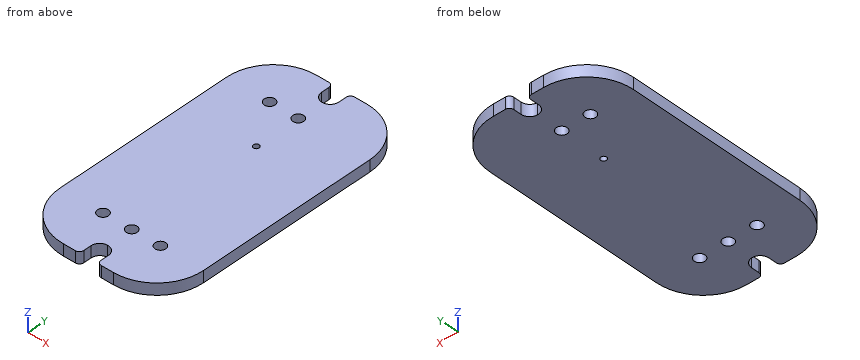
```python
from build123d import *

# Parameters (mm, degrees)
BOARD_DEPTH            = 0.8
SKETCH2_R              = 0.375
NON_PLATED_HOLES_DEPTH = 11.765221781
SKETCH3_R              = 0.2
PLATED_HOLES_DEPTH     = 11.765221781


with BuildPart() as part:
    # Sketch1 → BOARD (new body)
    with BuildSketch(Plane.XY):
        with BuildLine():
            Line((-0.6, 8.65), (-0.6, 9.2))
            ThreePointArc((-0.6, 9.2), (-0.687867966, 9.412132034), (-0.9, 9.5))
            Line((-0.9, 9.5), (-1.75, 9.5))
            ThreePointArc((-1.75, 9.5), (-4.048097039, 8.548097039), (-5, 6.25))
            Line((-5, 6.25), (-5, -6.25))
            ThreePointArc((-5, -6.25), (-4.048097039, -8.548097039), (-1.75, -9.5))
            Line((-1.75, -9.5), (-0.9, -9.5))
            ThreePointArc((-0.9, -9.5), (-0.687867966, -9.412132034), (-0.6, -9.2))
            Line((-0.6, -9.2), (-0.6, -8.65))
            ThreePointArc((-0.6, -8.65), (-0.424264069, -8.225735931), (0, -8.05))
            ThreePointArc((0, -8.05), (0.424264069, -8.225735931), (0.6, -8.65))
            Line((0.6, -8.65), (0.6, -9.2))
            ThreePointArc((0.6, -9.2), (0.687867966, -9.412132034), (0.9, -9.5))
            Line((0.9, -9.5), (1.75, -9.5))
            ThreePointArc((1.75, -9.5), (4.048097039, -8.548097039), (5, -6.25))
            Line((5, -6.25), (5, 6.25))
            ThreePointArc((5, 6.25), (4.048097039, 8.548097039), (1.75, 9.5))
            Line((1.75, 9.5), (0.9, 9.5))
            ThreePointArc((0.9, 9.5), (0.687867966, 9.412132034), (0.6, 9.2))
            Line((0.6, 9.2), (0.6, 8.65))
            ThreePointArc((0.6, 8.65), (0.424264069, 8.225735931), (0, 8.05))
            ThreePointArc((0, 8.05), (-0.424264069, 8.225735931), (-0.6, 8.65))
        make_face()
    extrude(amount=BOARD_DEPTH)

    # Sketch2 → NON-PLATED HOLES (cut, through all)
    with BuildSketch(Plane.XY):
        with Locations((2, -6.25)):
            Circle(SKETCH2_R)
        with Locations((0, -6.25)):
            Circle(SKETCH2_R)
        with Locations((-2, -6.25)):
            Circle(SKETCH2_R)
        with Locations((-2, 6.25)):
            Circle(SKETCH2_R)
        with Locations((0, 6.25)):
            Circle(SKETCH2_R)
    extrude(amount=NON_PLATED_HOLES_DEPTH, mode=Mode.SUBTRACT)

    # Sketch3 → PLATED HOLES (cut, through all)
    with BuildSketch(Plane.XY):
        with Locations((0, 3.1)):
            Circle(SKETCH3_R)
    extrude(amount=PLATED_HOLES_DEPTH, mode=Mode.SUBTRACT)


solid = part.part
```
Input: part model. Units: mm. Frame: model coordinates. Round coordinates to 2 decimals unless told otherwise and drop trailing zeros. Loops run counter-clockwise (first coordinate to the right, second up) from the corner with the lowest first, then second, coordinate; pieces in that order, holes last. Notation, with made-up numbers: (21.5, 27) -> (59.5, 27) arc R32 ccw to (59.5, 62) -> close; hole circle Ø1 at (9, -17.75). An arc over 180 degrees is marked (long way). Write each question's results on one line, items separated by ' | '.
1. Section B-B (x = 2). Return loops of the section in (y, z) (3 decimals), and give its area (3 significant figures).
Geometry results:
outline: (-9.49, 0) -> (-6.625, 0) -> (-6.625, 0.8) -> (-9.49, 0.8) -> close; (-5.875, 0) -> (9.49, 0) -> (9.49, 0.8) -> (-5.875, 0.8) -> close | area: 14.6 mm2
2. Section D-D (x = -2). Return loops of the section in (y, z) (3 decimals), and give its area (3 significant figures).
Geometry results:
outline: (-9.49, 0) -> (-6.625, 0) -> (-6.625, 0.8) -> (-9.49, 0.8) -> close; (-5.875, 0) -> (5.875, 0) -> (5.875, 0.8) -> (-5.875, 0.8) -> close; (6.625, 0) -> (9.49, 0) -> (9.49, 0.8) -> (6.625, 0.8) -> close | area: 14.0 mm2
3. Ray query, line 1 (X direction, y = -6.25, z = 0.35) (3 decimals); line 2 (Y direction, x = -0.25, z = 0.1); line 3 (X direction, y = 8.5, z = 0.1). Return the intervals inside material, ascending. Write a range as from..to.
Geometry results:
line 1: -5..-2.375, -1.625..-0.375, 0.375..1.625, 2.375..5 | line 2: -8.1..-6.53, -5.97..5.97, 6.53..8.1 | line 3: -4.1..-0.58, 0.58..4.1
4. Section A-A (y = 3.1). Return loops of the section in (x, z), and give its area (3 significant figures).
Geometry results:
outline: (-5, 0) -> (-0.2, 0) -> (-0.2, 0.8) -> (-5, 0.8) -> close; (0.2, 0) -> (5, 0) -> (5, 0.8) -> (0.2, 0.8) -> close | area: 7.68 mm2
5. First-contact query: P1, Ø5, axis at x = -2.5, y = 3.5, coming from the -Z side. Flat tip, straight axial feed; report the tip coordinate or a pass-through.
Geometry results:
P1: z = 0
6. Section C-C (z = 0.3). Return loops of the section in (x, y) (3 decimals).
Geometry results:
outline: (-5, -6.25) arc R3.25 ccw to (-1.75, -9.5) -> (-0.9, -9.5) arc R0.3 ccw to (-0.6, -9.2) -> (-0.6, -8.65) arc R0.6 cw to (0.6, -8.65) -> (0.6, -9.2) arc R0.3 ccw to (0.9, -9.5) -> (1.75, -9.5) arc R3.25 ccw to (5, -6.25) -> (5, 6.25) arc R3.25 ccw to (1.75, 9.5) -> (0.9, 9.5) arc R0.3 ccw to (0.6, 9.2) -> (0.6, 8.65) arc R0.6 cw to (-0.6, 8.65) -> (-0.6, 9.2) arc R0.3 ccw to (-0.9, 9.5) -> (-1.75, 9.5) arc R3.25 ccw to (-5, 6.25) -> close; hole circle Ø0.75 at (-2, -6.25); hole circle Ø0.75 at (-2, 6.25); hole circle Ø0.75 at (0, -6.25); hole circle Ø0.75 at (0, 6.25); hole circle Ø0.4 at (0, 3.1); hole circle Ø0.75 at (2, -6.25)
